```python
from build123d import *

# Parameters (mm, degrees)
BOSS_EXTRUDE1_DEPTH = 4
SKETCH2_R           = 2.2
CUT_EXTRUDE1_DEPTH  = 1000
FILLET1_R           = 3
MIRROR2_OUTLINE_R   = 2.2
MIRROR2_DEPTH       = 4
FILLET4_R           = 120


# Read off the part's stored shape, not the designer's step: Mirror2
with BuildPart() as part:
    # Sketch1 → Boss-Extrude1 (new body)
    with BuildSketch(Plane(origin=(0, 0, 0), x_dir=(1, 0, 0), z_dir=(0, 1, 0))):
        Polygon((0, 0), (60, 0), (60, 13.5), (56.456743563, 71.5), (37.872574787, 91.086440997), (0, 102.307763512), align=None)
    extrude(amount=BOSS_EXTRUDE1_DEPTH)

    # Sketch2 → Cut-Extrude1 (cut)
    with BuildSketch(Plane(origin=(0, 4, 0), x_dir=(1, 0, 0), z_dir=(0, 1, 0))):
        with Locations(Location((39.912815741, 81.236064514, 0), (0, 0, 270))):
            Circle(SKETCH2_R)
        with Locations(Location((54.7, 4.95, 0), (0, 0, 270))):
            Circle(SKETCH2_R)
        with Locations(Location((31.280273227, 73.045264202, 0), (0, 0, 270))):
            Circle(SKETCH2_R)
        with Locations(Location((42.8, 4.95, 0), (0, 0, 270))):
            Circle(SKETCH2_R)
        with Locations(Location((38.094468445, 65.86356917, 0), (0, 0, 270))):
            Circle(SKETCH2_R)
        with Locations(Location((46.727010958, 74.054369482, 0), (0, 0, 270))):
            Circle(SKETCH2_R)
        with BuildLine():
            Line((56.513876684, 21.365861695), (54.367510102, 56.5))
            ThreePointArc((54.367510102, 56.5), (51.361917218, 59.505592884), (48.356324334, 56.5))
            Line((48.356324334, 56.5), (50.547392357, 20.634138305))
            ThreePointArc((50.547392357, 20.634138305), (53.896496216, 18.016757837), (56.513876684, 21.365861695))
        make_face()
    extrude(amount=-CUT_EXTRUDE1_DEPTH, mode=Mode.SUBTRACT)

    # Fillet1
    # the kernel refuses this fillet: 3 mm, written as the material it takes off along each edge
    with BuildSketch(Plane(origin=(56.456743563, -2.729776757, -71.5), x_dir=(0.060976949232979236, 0, 0.99813917449534), z_dir=(0, 1, 0))) as fillet1_piece_1:
        with BuildLine():
            CenterArc((FILLET1_R * 0.363970234266, -FILLET1_R), FILLET1_R, 90, 40)
            Line((-FILLET1_R * 0.27881737542, -FILLET1_R * 0.233955556881), (0, 0))
            Line((0, 0), (FILLET1_R * 0.363970234266, 0))
        make_face()
    extrude(amount=9.459553514, mode=Mode.SUBTRACT)
    with BuildSketch(Plane(origin=(60, -0.228876509, -13.5), x_dir=(0, 0, 1), z_dir=(0, 1, 0))) as fillet1_piece_2:
        with BuildLine():
            CenterArc((FILLET1_R * 0.0305168678995, -FILLET1_R), FILLET1_R, 90, 3.495890522)
            Line((-FILLET1_R * 0.0304600813334, -FILLET1_R * 0.00186082550466), (0, 0))
            Line((0, 0), (FILLET1_R * 0.0305168678995, 0))
        make_face()
    extrude(amount=4.457753018, mode=Mode.SUBTRACT)

    # Mirror2 outline → Mirror2 (add)
    with BuildSketch(Plane(origin=(0, 0, 0), x_dir=(1, 0, 0), z_dir=(0, 1, 0))):
        with BuildLine():
            Line((60, -13.408449396), (60, 0))
            Line((60, 0), (0, 0))
            Line((0, 0), (0, 102.307763512))
            Line((0, 102.307763512), (-37.872574787, 91.086440997))
            Line((-37.872574787, 91.086440997), (-55.705178644, 72.292097946))
            ThreePointArc((-55.705178644, 72.292097946), (-56.280173438, 71.423240183), (-56.523324946, 70.410121152))
            Line((-56.523324946, 70.410121152), (-59.994417523, 13.591380244))
            ThreePointArc((-59.994417523, 13.591380244), (-59.998604056, 13.4999574), (-60, 13.408449396))
            Line((-60, 13.408449396), (-60, -13.408449396))
            ThreePointArc((-60, -13.408449396), (-59.998604056, -13.4999574), (-59.994417523, -13.591380244))
            Line((-59.994417523, -13.591380244), (-56.523324946, -70.410121152))
            ThreePointArc((-56.523324946, -70.410121152), (-56.280173438, -71.423240183), (-55.705178644, -72.292097946))
            Line((-55.705178644, -72.292097946), (-37.872574787, -91.086440997))
            Line((-37.872574787, -91.086440997), (0, -102.307763512))
            Line((0, -102.307763512), (37.872574787, -91.086440997))
            Line((37.872574787, -91.086440997), (55.705178644, -72.292097946))
            ThreePointArc((55.705178644, -72.292097946), (56.280173438, -71.423240183), (56.523324946, -70.410121152))
            Line((56.523324946, -70.410121152), (59.994417523, -13.591380244))
            ThreePointArc((59.994417523, -13.591380244), (59.998604056, -13.4999574), (60, -13.408449396))
        make_face()
        with Locations((-39.912815741, -81.236064514)):
            Circle(MIRROR2_OUTLINE_R, mode=Mode.SUBTRACT)
        with Locations((-46.727010958, -74.054369482)):
            Circle(MIRROR2_OUTLINE_R, mode=Mode.SUBTRACT)
        with Locations((-38.094468445, -65.86356917)):
            Circle(MIRROR2_OUTLINE_R, mode=Mode.SUBTRACT)
        with Locations((-31.280273227, -73.045264202)):
            Circle(MIRROR2_OUTLINE_R, mode=Mode.SUBTRACT)
        with BuildLine():
            ThreePointArc((-48.356324334, -56.5), (-51.361917218, -59.505592884), (-54.367510102, -56.5))
            Line((-54.367510102, -56.5), (-56.513876684, -21.365861695))
            ThreePointArc((-56.513876684, -21.365861695), (-53.896496215, -18.016757837), (-50.547392357, -20.634138305))
            Line((-50.547392357, -20.634138305), (-48.356324334, -56.5))
        make_face(mode=Mode.SUBTRACT)
        with Locations((-54.7, -4.95)):
            Circle(MIRROR2_OUTLINE_R, mode=Mode.SUBTRACT)
        with Locations((-42.8, -4.95)):
            Circle(MIRROR2_OUTLINE_R, mode=Mode.SUBTRACT)
        with Locations((39.912815741, -81.236064514)):
            Circle(MIRROR2_OUTLINE_R, mode=Mode.SUBTRACT)
        with Locations((31.280273227, -73.045264202)):
            Circle(MIRROR2_OUTLINE_R, mode=Mode.SUBTRACT)
        with Locations((38.094468445, -65.86356917)):
            Circle(MIRROR2_OUTLINE_R, mode=Mode.SUBTRACT)
        with Locations((46.727010958, -74.054369482)):
            Circle(MIRROR2_OUTLINE_R, mode=Mode.SUBTRACT)
        with BuildLine():
            ThreePointArc((54.367510102, -56.5), (51.361917218, -59.505592884), (48.356324334, -56.5))
            Line((48.356324334, -56.5), (50.547392357, -20.634138305))
            ThreePointArc((50.547392357, -20.634138305), (53.896496215, -18.016757837), (56.513876684, -21.365861695))
            Line((56.513876684, -21.365861695), (54.367510102, -56.5))
        make_face(mode=Mode.SUBTRACT)
        with Locations((42.8, -4.95)):
            Circle(MIRROR2_OUTLINE_R, mode=Mode.SUBTRACT)
        with Locations((54.7, -4.95)):
            Circle(MIRROR2_OUTLINE_R, mode=Mode.SUBTRACT)
        with Locations((-54.7, 4.95)):
            Circle(MIRROR2_OUTLINE_R, mode=Mode.SUBTRACT)
        with Locations((-42.8, 4.95)):
            Circle(MIRROR2_OUTLINE_R, mode=Mode.SUBTRACT)
        with BuildLine():
            ThreePointArc((-54.367510102, 56.5), (-51.361917218, 59.505592884), (-48.356324334, 56.5))
            Line((-48.356324334, 56.5), (-50.547392357, 20.634138305))
            ThreePointArc((-50.547392357, 20.634138305), (-53.896496215, 18.016757837), (-56.513876684, 21.365861695))
            Line((-56.513876684, 21.365861695), (-54.367510102, 56.5))
        make_face(mode=Mode.SUBTRACT)
        with Locations((-46.727010958, 74.054369482)):
            Circle(MIRROR2_OUTLINE_R, mode=Mode.SUBTRACT)
        with Locations((-38.094468445, 65.86356917)):
            Circle(MIRROR2_OUTLINE_R, mode=Mode.SUBTRACT)
        with Locations((-31.280273227, 73.045264202)):
            Circle(MIRROR2_OUTLINE_R, mode=Mode.SUBTRACT)
        with Locations((-39.912815741, 81.236064514)):
            Circle(MIRROR2_OUTLINE_R, mode=Mode.SUBTRACT)
    extrude(amount=MIRROR2_DEPTH)

    # Fillet4
    fillet4_edges = [part.edges().sort_by_distance(p)[0] for p in [
        (0, 2, 102.307763512),
        (0, 2, -102.307763512),
    ]]
    fillet(fillet4_edges, radius=FILLET4_R)


solid = part.part
```
Work out the finished part from the listing and answer in its coordinate system (mm). A direction names the side the tool comes from. Give positions to 0.01 mm unless a question says otherwise; leave off trailing zeros. Order: outer loops, then holes, each group sorted by start corner. A loop starts at its lowest first (then second) coordinate and runs counter-clockwise, first axis right, second up.
1. Each of these flat-tipped pins is pushed along its axis until it touches: P1, Ø5, axis at x = -42.8, z = -4.95, coming from the +Y side; P2, Ø2, axis at y = 0.5, z = -41, coming from the -X side. Where does it stop, or does it pass through?
Result sheet:
P1: stops at y = 4
P2: stops at x = -58.38
2. Section C-C, the plane y = 1.3 is taken. Give the number of separate pieces and of enclosed holes in the cut face, and give its area (3 significant figures).
Result sheet:
separate pieces: 1
enclosed holes: 28
area: 19,700 mm2
3. Section B-B, the plane z = -53 is taken. Determine the outline of the cut face in (x, y), and give its area (3 significant figures).
Result sheet:
outline: (-57.59, 0) - (-54.58, 0) - (-54.58, 4) - (-57.59, 4) - close; (-48.57, 0) - (48.57, 0) - (48.57, 4) - (-48.57, 4) - close; (54.58, 0) - (57.59, 0) - (57.59, 4) - (54.58, 4) - close
area: 413 mm2
4. For faces 1 (the flat face through (60, 2, 0)), 2 (the flat face through (-55.426, 1.972, 39.179)), determine the directions among +Z, -Z, +X, -X, +Y, -Y from which every point of the face is accessible in a straight line to the end or side of a thin tool.
Result sheet:
face 1: +Z, -Z, +X, +Y, -Y
face 2: +Y, -Y
5. Straight lines are drawn through the part: L1, parallel to X at y = 1.5, z = 4.95; L2, parallel to X at y = 2.6, z = 51; L3, parallel to X at y = 0.25, z = -33. For each, find the intervals that lie inside material, in ascending order.
Result sheet:
L1: x = -60 to -56.9, -52.5 to -45, -40.6 to 40.6, 45 to 52.5, 56.9 to 60
L2: x = -57.71 to -54.7, -48.69 to 48.69, 54.7 to 57.71
L3: x = -58.81 to -55.8, -49.79 to 49.79, 55.8 to 58.81
6. Section D-D, the plane x = -23 is taken. Determine the outline of the cut face in (y, z), and give its area (3 significant figures).
Result sheet:
outline: (0, -94.93) - (4, -94.93) - (4, 94.93) - (0, 94.93) - close
area: 759 mm2
7. The mould has two halves that part along X. Classify faces 3 (the cylindrical face through (-31.567, 1.972, -75.227)), 4 (the flat face through (46.91, 1.97, -81.56)), 5 (the flat face through (-46.91, 1.97, 81.56)): released by +X, released by -X, zero draft, split by the parting line, or undercut.
Result sheet:
face 3: undercut
face 4: released by +X
face 5: released by -X
8. Section A-A, the plane z = 4.95 is taken. Determine the outline of the cut face in (x, y).
Result sheet:
outline: (-60, 0) - (-56.9, 0) - (-56.9, 4) - (-60, 4) - close; (-52.5, 0) - (-45, 0) - (-45, 4) - (-52.5, 4) - close; (-40.6, 0) - (40.6, 0) - (40.6, 4) - (-40.6, 4) - close; (45, 0) - (52.5, 0) - (52.5, 4) - (45, 4) - close; (56.9, 0) - (60, 0) - (60, 4) - (56.9, 4) - close
